Verification items for the finished model (mm, model axes). Face numbers are marked on the shaded views. A direction names the side the tool comes from. Coordinates: 2 decimals unless noted, no trailing zeros. Order: outer loops, then holes, each group sorted by start corner. A loop starts at its lowest first (then second) coordinate and runs counter-clockwise, first axis right, second up. Notation, with made-up numbers: (-37.5, -13) -> (-27.5, -13) arc R12 cw to (-27.5, -1) -> close; hole circle Ø10 at (52.25, -27). An arc over 180 degrees is marked (long way). Use CSV: the item, a comma, the result in double quotes. Start each with the question number.
1) Sectioned sample at A-A on y = 1. Record the boundary of the cut face in (x, z) (1 decimal), then the cut area to 3 significant figures.
2) Scan lines: line 1 along X through (y, z) = (1.9, 35) (3 decimals); line 2 along Y through (x, z) = (1, -18) (3 decimals); line 3 along X through (y, z) = (1.65, 5) (3 decimals). Record each from-to range of solid material in increasing order.
3) Tool access check on the marked faces 1 and 2. Record the directions out of +Z, -Z, +X, -X, +Y, -Y that give a thin tool (end or side, any length) a straight path to the whole face; none if there is none.
4) Sectioned sample at C-C on y = 4.25. Record the boundary of the cut face in (x, z).
5) Sectioned sample at B-B on z = 19. Record the boundary of the cut face in (x, y) (3 decimals), then the cut area to 3 significant figures.
6) Go/stop test with flat-tipped pins: pin 1 (1.9 mm diameter, centred on x = -7.74, z = 5, fed in from -Y); pin 2 (5.5 mm diameter, centred on x = -6.5, z = -2.5, fed in from +Y) (3 decimals); pin 3 (2.5 mm diameter, centred on y = 1, z = 25, fed in from +X) (3 decimals); pin 4 (1.6 mm diameter, centred on y = 1.5, z = 16, fed in from +X). Record where each tip stops, or that it passes through.
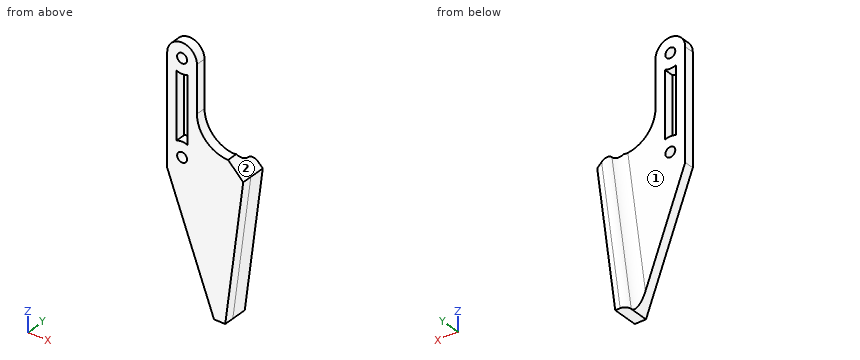
from build123d import *

# Parameters (mm, degrees)
CROQUIS1_R              = 1.5875
SALIENTE_EXTRUIR1_DEPTH = 3.175
CORTAR_EXTRUIR1_DEPTH   = 3.175
CORTAR_EXTRUIR3_DEPTH   = 10
CORTAR_EXTRUIR8_DEPTH   = 10
BOSS_EXTRU_1_DEPTH      = 5
CONG_1_R                = 2
CONG_2_R                = 3


with BuildPart() as part:
    # Croquis1 → Saliente-Extruir1 (new body)
    with BuildSketch(Plane(origin=(0, 0, 0), x_dir=(1, 0, 0), z_dir=(0, 1, 0))):
        with BuildLine():
            Line((-12.5, 0), (-12.5, -40))
            Line((-12.5, -40), (-2.975, -40))
            Line((-2.975, -40), (-2.975, -20))
            ThreePointArc((-2.975, -20), (-0.046067812, -12.928932188), (7.025, -10))
            Line((7.025, -10), (12.5, -10))
            Line((12.5, -10), (12.5, 40))
            Line((12.5, 40), (2.5, 40))
            Line((2.5, 40), (-12.5, 0))
        make_face()
        with Locations(Location((-7.7375, -5, 0), (0, 0, 270))):
            Circle(CROQUIS1_R, mode=Mode.SUBTRACT)
        with Locations(Location((-7.7375, -35, 0), (0, 0, 270))):
            Circle(CROQUIS1_R, mode=Mode.SUBTRACT)
    extrude(amount=SALIENTE_EXTRUIR1_DEPTH)

    # Croquis2 → Cortar-Extruir1 (cut)
    with BuildSketch(Plane(origin=(0, 3.175, 0), x_dir=(1, 0, 0), z_dir=(0, 1, 0))):
        Polygon((12.5, -10), (6.1, 40), (12.5, 40), align=None)
    extrude(amount=-CORTAR_EXTRUIR1_DEPTH, mode=Mode.SUBTRACT)

    # Croquis3 → Cortar-Extruir3 (cut)
    with BuildSketch(Plane(origin=(0, 3.175, 0), x_dir=(1, 0, 0), z_dir=(0, 1, 0))):
        with BuildLine():
            ThreePointArc((-5.975, -30.575635639), (-7.7375, -30.2375), (-9.5, -30.575635639))
            Line((-9.5, -30.575635639), (-9.5, -9.427055314))
            ThreePointArc((-9.5, -9.427055314), (-7.7375, -9.765), (-5.975, -9.427055314))
            Line((-5.975, -9.427055314), (-5.975, -14.803847577))
            Line((-5.975, -14.803847577), (-5.975, -30.575635639))
        make_face()
        with BuildLine():
            ThreePointArc((-12.5, -35), (-7.7375, -39.7625), (-2.975, -35))
            Line((-2.975, -35), (-2.975, -40))
            Line((-2.975, -40), (-12.5, -40))
            Line((-12.5, -40), (-12.5, -35))
        make_face()
    extrude(amount=-CORTAR_EXTRUIR3_DEPTH, mode=Mode.SUBTRACT)

    # Croquis5 → Cortar-Extruir8 (cut)
    with BuildSketch(Plane(origin=(0, 3.175, 0), x_dir=(1, 0, 0), z_dir=(0, 1, 0))):
        Polygon((7.025, -10), (11.878723404, -5.146276596), (12.5, -10), align=None)
    extrude(amount=-CORTAR_EXTRUIR8_DEPTH, mode=Mode.SUBTRACT)

    # Esquisse1 → Boss.-Extru.1 (add)
    with BuildSketch(Plane(origin=(0, 3.175, 0), x_dir=(1, 0, 0), z_dir=(0, 1, 0))):
        Polygon((11.878723404, -5.146276596), (6.1, 40), (2.5, 40), (8.687234043, -8.337765957), align=None)
    extrude(amount=BOSS_EXTRU_1_DEPTH)

    # Congé1
    cong_1_edges = [part.edges().sort_by_distance(p)[0] for p in [
        (5.593617021, 8.175, -15.831117021),
    ]]
    fillet(cong_1_edges, radius=CONG_1_R)

    # Congé2
    cong_2_edges = [part.edges().sort_by_distance(p)[0] for p in [
        (5.593617021, 3.175, -15.831117021),
    ]]
    fillet(cong_2_edges, radius=CONG_2_R - 0.0001)  # a hair under: the kernel refuses the full size


solid = part.part
Answers follow:
1,outline,"(-12.5, 0) -> (2.5, -40) -> (6.1, -40) -> (11.9, 5.1) -> (7, 10) arc R10 cw to (-3, 20) -> (-3, 35) arc R4.8 ccw to (-12.5, 35) -> close; hole (-9.5, 9.4) arc R4.8 cw to (-6, 9.4) -> (-6, 30.6) arc R4.8 cw to (-9.5, 30.6) -> close; hole circle Ø3.2 at (-7.7, 5); hole circle Ø3.2 at (-7.7, 35)"
1,area,"983 mm²"
2,line 1,"x = -12.5 to -9.325, -6.15 to -2.975"
2,line 2,"y = 0 to 3.175"
2,line 3,"x = -12.5 to -9.325, -6.15 to 11.86"
3,face 1,"+Z, -X, +Y"
3,face 2,"+Z, +X, +Y, -Y"
4,outline,"(1.97, -38.6) -> (2.5, -40) -> (6.1, -40) -> (11.88, 5.15) -> (8.06, 8.96) -> close"
5,outline,"(-12.5, 0) -> (-9.5, 0) -> (-9.5, 3.175) -> (-12.5, 3.175) -> close; (-5.975, 0) -> (-2.925, 0) -> (-2.925, 3.175) -> (-5.975, 3.175) -> close"
5,area,"19.2 mm²"
6,pin 1,"passes through"
6,pin 2,"stops at y = 3.175"
6,pin 3,"stops at x = -2.975"
6,pin 4,"stops at x = -1.75"
